Input: part model. Units: mm. Frame: model coordinates. Face numbers are marked on the shaded views. A direction names the side the tool comes from. Coordinates: 2 decimals unless noted, no trailing zeros. Write each loop counter-clockwise with the first axis right and the second up, starting at its lowest first coordinate (ties: lowest second). Pieces come first, ordered by that corner, then holes. Notation, with made-up numbers: (64, 1.25) - (95, 1.25) arc R20 ccw to (95, 23.25) - close; hole circle Ø5 at (28.5, -9.75). An arc over 180 degrees is marked (long way). Use a Markdown table: item, result. Add a question column.
Q1. Section query D-D (x = -1.75). Return the cut outline in (y, z), then the cut area to 3 significant figures.
Q2. Pin query (flat end, axial travel): P1, Ø1.5, axis at y = -0.5, z = 3.5, coming from the +X side; P2, Ø1, axis at x = -2, z = 3.5, coming from the +Y side; P3, Ø5, axis at x = 0.5, y = 3, coming from the -Z side. Return the tip coordinate at first contact, or that it passes through.
Q3. Mould query, pull axis Z, two halves, no side actions, for the marked faces 1, 2 and 3. Classes: released by +Z, released by -Z, zero draft, split by the parting line, or undercut.
Q4. Set-up query: the marked faces 4 and 5. Return all of +Z, -Z, +X, -X, +Y, -Y with unobstructed straight access to the full face (end or side cutting, diameter ignored); none if empty.
Q5. Section query C-C (x = 2.5). Return the cut outline in (y, z), then the cut area to 3 significant figures.
Q6. Section query A-A (z = 0). Return the cut outline in (x, y).
Q7. Material intervals for probe 1 along Y at (x, z) = (-2.5, 0); probe 2 along Z at (x, y) = (-3.5, -0.25); probe 3 along Z at (x, y) = (3.25, 0), sorted ascending. Write a range as from..to.
from build123d import *

# Parameters (mm, degrees)
FILLET1_R     = 0.15
FILLET2_R     = 0.15
CHAMFER1_SIZE = 0.2


with BuildPart() as part:
    # Sketch1 → Revolve1 (revolve)
    with BuildSketch(Plane.XY):
        Polygon((0, 12.95), (0, 8), (-5.5, 8), (-5.5, 6.1), (6.4, 6.1), (6.4, 12.95), align=None)
    revolve(axis=Axis((6.4, 0, 0), (-1, 0, 0)))

    # Fillet1
    fillet1_edges = [part.edges().sort_by_distance(p)[0] for p in [
        (0, -12.95, 0),
        (6.4, -12.95, 0),
    ]]
    fillet(fillet1_edges, radius=FILLET1_R)

    # Fillet2
    fillet2_edges = [part.edges().sort_by_distance(p)[0] for p in [
        (6.4, -6.1, 0),
    ]]
    fillet(fillet2_edges, radius=FILLET2_R)

    # Chamfer1
    chamfer1_edges = [part.edges().sort_by_distance(p)[0] for p in [
        (-5.5, -6.1, 0),
        (-5.5, -8, 0),
    ]]
    chamfer(chamfer1_edges, length=CHAMFER1_SIZE)


solid = part.part
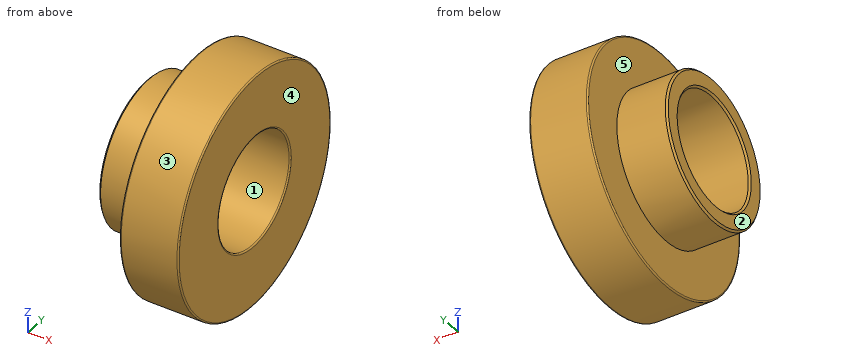
Values follow:
| question | item | result |
|---|---|---|
| 1 | outline | circle Ø16 at (0, 0); hole circle Ø12.2 at (0, 0) |
| 1 | area | 84.2 mm2 |
| 2 | P1 | through |
| 2 | P2 | y = 7.42 |
| 2 | P3 | z = -12.94 |
| 3 | face 1 | undercut |
| 3 | face 2 | zero draft |
| 3 | face 3 | split by the parting line |
| 4 | face 4 | +Z, -Z, +X, +Y, -Y |
| 4 | face 5 | -X |
| 5 | outline | circle Ø25.9 at (0, 0); hole circle Ø12.2 at (0, 0) |
| 5 | area | 410 mm2 |
| 6 | outline | (-5.5, -7.8) - (-5.3, -8) - (0, -8) - (0, -12.8) arc R0.15 ccw to (0.15, -12.95) - (6.25, -12.95) arc R0.15 ccw to (6.4, -12.8) - (6.4, -6.25) arc R0.15 ccw to (6.25, -6.1) - (-5.3, -6.1) - (-5.5, -6.3) - close; (-5.5, 6.3) - (-5.3, 6.1) - (6.25, 6.1) arc R0.15 ccw to (6.4, 6.25) - (6.4, 12.8) arc R0.15 ccw to (6.25, 12.95) - (0.15, 12.95) arc R0.15 ccw to (0, 12.8) - (0, 8) - (-5.3, 8) - (-5.5, 7.8) - close |
| 7 | probe 1 | -8..-6.1, 6.1..8 |
| 7 | probe 2 | -8..-6.09, 6.09..8 |
| 7 | probe 3 | -12.95..-6.1, 6.1..12.95 |
